```python
from build123d import *

# Parameters (mm, degrees)
PAD_DEPTH    = 6
SKETCH001_R  = 1.5
HOLE_DEPTH   = 25
FILLET_R     = 0.25
CHAMFER_SIZE = 0.2


with BuildPart() as part:
    # Sketch → Pad (new body)
    with BuildSketch(Plane.YZ):
        Polygon((-13, 0.5), (-13, -1.5), (13, -1.5), (13, 0.5), (12.5, 0.5), (12.5, 2e-06), (12, 2e-06), (12, 0.5), (11.5, 0.5), (11.5, 0), (11, 0), (11, 0.5), (10.5, 0.5), (10.5, 0), (10, 0), (10, 0.5), (9.5, 0.5), (9.5, 0), (9, 0), (9, 0.5), (8.5, 0.5), (8.5, 0), (8, 0), (8, 0.5), (7.5, 0.5), (7.5, 0), (7, 0), (7, 0.5), (6.5, 0.5), (6.5, 0), (0, 0), (-6.5, 0), (-6.5, 0.5), (-7, 0.5), (-7, 0), (-7.5, 0), (-7.5, 0.5), (-8, 0.5), (-8, 0), (-8.5, 0), (-8.5, 0.5), (-9, 0.5), (-9, 0), (-9.5, 0), (-9.5, 0.5), (-10, 0.5), (-10, 0), (-10.5, 0), (-10.5, 0.5), (-11, 0.5), (-11, 0), (-11.5, 0), (-11.5, 0.5), (-12, 0.5), (-12, 0), (-12.5, 0), (-12.5, 0.5), align=None)
    extrude(amount=PAD_DEPTH)

    # Sketch001 (on Face58 of Pad) → Hole (cut)
    with BuildSketch(Plane(origin=(0, 0, 0), x_dir=(0, -1, 0), z_dir=(0, 0, 1))):
        with Locations((0, 3)):
            Circle(SKETCH001_R)
    extrude(amount=-HOLE_DEPTH, mode=Mode.SUBTRACT)

    # Fillet
    fillet_edges = [part.edges().sort_by_distance(p)[0] for p in [
        (3, -1.5, 0),
        (3, -1.5, -1.5),
    ]]
    fillet(fillet_edges, radius=FILLET_R)

    # Chamfer
    chamfer_edges = [part.edges().sort_by_distance(p)[0] for p in [
        (3, -13, 0.5),
        (3, -12, 0.5),
        (3, -12.5, 0.5),
        (3, -11.5, 0.5),
        (3, -11, 0.5),
        (3, -10.5, 0.5),
        (3, -10, 0.5),
        (3, -9.5, 0.5),
        (3, -9, 0.5),
        (3, -8.5, 0.5),
        (3, -8, 0.5),
        (3, -7.5, 0.5),
        (3, -7, 0.5),
        (3, -6.5, 0.5),
        (3, 6.5, 0.5),
        (3, 7, 0.5),
        (3, 7.5, 0.5),
        (3, 8, 0.5),
        (3, 8.5, 0.5),
        (3, 9, 0.5),
        (3, 9.5, 0.5),
        (3, 10, 0.5),
        (3, 10.5, 0.5),
        (3, 11, 0.5),
        (3, 11.5, 0.5),
        (3, 12, 0.5),
        (3, 12.5, 0.5),
        (3, 13, 0.5),
    ]]
    chamfer(chamfer_edges, length=CHAMFER_SIZE)


solid = part.part
```
Verification items for the finished model (mm, model axes). Coordinates: 2 decimals unless noted, no trailing zeros. Loops run counter-clockwise (first coordinate to the right, second up) from the corner with the lowest first, then second, coordinate; pieces in that order, holes last. Notation, with made-up numbers: (-38.75, -7.75) -> (-34.75, -7.75) arc R12 ccw to (-34.75, 15.25) -> close; hole circle Ø7 at (5.25, -6.5). An arc over 180 degrees is marked (long way). Answer in a Markdown table with one row per item. Add a question column.
1. Section check A-A, the plane y = 0. Enter the section's corners in (x, z), then the cut area to 3 significant figures.
2. Material ranges on probe 1 along X at (y, z) = (0, -0.85); probe 2 along Z at (x, y) = (3, 3); probe 3 along Y at (x, z) = (2.45, -1.1), recorded low to high. Write a range as [from, to].
3. Depth check by flat-ended pin: P1, Ø1.5, axis at x = 2, y = 3, coming from the +Z side. Enter the tip coordinate at first touch or a pass-through.
4. Section check B-B, the plane z = -1. Enter the section's corners in (x, y), then the cut area to 3 significant figures.
5. Draft check along Y on faces 1 (the face through (3, -13, -1)), 2 (the face through (2, 2, 0)), 3 (the face through (0, 0, -1)). Enter one of: +Y half, -Y half, draft (parallel to the pull), parting line (faces both ways), or undercut.
Derived:
| question | item | result |
|---|---|---|
| 1 | outline | (0, -1.5) -> (1.25, -1.5) arc R0.25 ccw to (1.5, -1.25) -> (1.5, -0.25) arc R0.25 ccw to (1.25, 0) -> (0, 0) -> close; (4.5, -1.25) arc R0.25 ccw to (4.75, -1.5) -> (6, -1.5) -> (6, 0) -> (4.75, 0) arc R0.25 ccw to (4.5, -0.25) -> close |
| 1 | area | 4.45 mm² |
| 2 | probe 1 | x = [0, 1.5], [4.5, 6] |
| 2 | probe 2 | z = [-1.5, 0] |
| 2 | probe 3 | y = [-13, -1.4], [1.4, 13] |
| 3 | P1 | stops at z = 0 |
| 4 | outline | (0, -13) -> (6, -13) -> (6, 13) -> (0, 13) -> close; hole circle Ø3 at (3, 0) |
| 4 | area | 149 mm² |
| 5 | face 1 | -Y half |
| 5 | face 2 | undercut |
| 5 | face 3 | draft |
